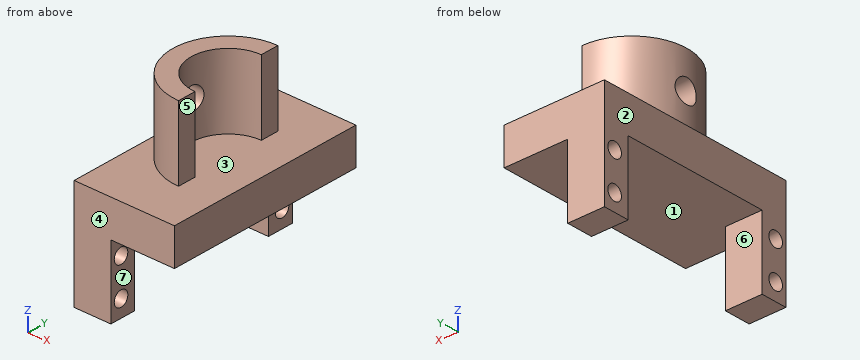
from build123d import *

# Parameters (mm, degrees)
BOSS_EXTRUDE1_DEPTH = 19.812
SKETCH2_R           = 3.175
CUT_EXTRUDE2_DEPTH  = 29.880704735
SKETCH3_W           = 34.1757
SKETCH3_H           = 54.2544
BOSS_EXTRUDE2_DEPTH = 9.906
SKETCH4_W           = 9.906
SKETCH4_H           = 7.112
BOSS_EXTRUDE3_DEPTH = 19.4691
SKETCH5_R           = 2.032
CUT_EXTRUDE3_DEPTH  = 53.599999528
SKETCH6_W           = 7.112
SKETCH6_H           = 54.2544
CUT_EXTRUDE4_DEPTH  = 44.715433515


with BuildPart() as part:
    # Sketch1 → Boss-Extrude1 (new body)
    with BuildSketch(Plane.XY):
        with BuildLine():
            Line((0, 14.859), (0, 9.906))
            ThreePointArc((0, 9.906), (-9.906, 0), (0, -9.906))
            Line((0, -9.906), (0, -14.859))
            ThreePointArc((0, -14.859), (-14.859, 0), (0, 14.859))
        make_face()
    extrude(amount=BOSS_EXTRUDE1_DEPTH)

    # Sketch2 → Cut-Extrude2 (cut, through all)
    with BuildSketch(Plane(origin=(0, 0, 0), x_dir=(0, 0, -1), z_dir=(1, 0, 0))):
        with Locations(Location((-9.906, 0, 0), (0, 0, 90))):
            Circle(SKETCH2_R)
    extrude(amount=-CUT_EXTRUDE2_DEPTH, mode=Mode.SUBTRACT)

    # Sketch3 → Boss-Extrude2 (add)
    with BuildSketch(Plane(origin=(0, 0, 0), x_dir=(-1, 0, 0), z_dir=(0, 0, -1))):
        Rectangle(SKETCH3_W, SKETCH3_H)
    extrude(amount=BOSS_EXTRUDE2_DEPTH)

    # Sketch4 → Boss-Extrude3 (add)
    with BuildSketch(Plane(origin=(0, 0, -9.906), x_dir=(-1, 0, 0), z_dir=(0, 0, -1))):
        with Locations((12.13485, -23.5712)):
            Rectangle(SKETCH4_W, SKETCH4_H)
        with Locations((12.13485, 23.5712)):
            Rectangle(SKETCH4_W, SKETCH4_H)
    extrude(amount=BOSS_EXTRUDE3_DEPTH)

    # Sketch5 → Cut-Extrude3 (cut, through all)
    with BuildSketch(Plane.ZY.offset(17.08785)):
        with Locations((-24.8031, 24.0792)):
            Circle(SKETCH5_R)
        with Locations((-14.8971, 24.0792)):
            Circle(SKETCH5_R)
        with Locations(Location((-14.8971, -24.0792, 0), (0, 0, 270))):
            Circle(SKETCH5_R)
        with Locations(Location((-24.8031, -24.0792, 0), (0, 0, 270))):
            Circle(SKETCH5_R)
    extrude(amount=-CUT_EXTRUDE3_DEPTH, mode=Mode.SUBTRACT)

    # Sketch6 → Cut-Extrude4 (cut, through all)
    with BuildSketch(Plane(origin=(0, 0, -9.906), x_dir=(-1, 0, 0), z_dir=(0, 0, -1))):
        with Locations((-13.53185, 0)):
            Rectangle(SKETCH6_W, SKETCH6_H)
    extrude(amount=-CUT_EXTRUDE4_DEPTH, mode=Mode.SUBTRACT)


solid = part.part
Verification items for the finished model (mm, model axes). Face numbers are marked on the shaded views. A direction names the side the tool comes from. Give positions to 0.01 mm unless a question says otherwise; leave off trailing zeros. Write each loop counter-clockwise with the first axis right and the second up, starting at its lowest first coordinate (ties: lowest second). Pieces come first, ordered by that corner, then holes. Notation, with made-up numbers: (75, 70.5) - (85, 70.5) arc R31 cw to (85, 96.5) - close; hole circle Ø7 at (76.5, 24.25). An arc over 180 degrees is marked (long way). Answer as CSV lines item,"result". Start each with the question number.
1. Depth check by flat-ended pin: pin 1 (8 mm diameter, centred on x = 3, y = 12.5, fed in from -Z); pin 2 (4 mm diameter, centred on y = -13, z = 6, fed in from +X); pin 3 (2 mm diameter, centred on y = 21.5, z = 0.5, fed in from +X); pin 4 (2 mm diameter, centred on x = 3, y = -20, fed in from +Z). Enter the tip coordinate at first touch or a pass-through.
2. Draft check along Y on the marked faces 1, 2, 3 and 4. Enter one of: pulls with the +Y half, pulls with the -Y half, needs draft (parallel to the pull), parting line crosses it, or undercut.
3. Sectioned sample at D-D (z = 8). Record the boundary of the cut face in (x, y).
4. Sectioned sample at A-A (y = 0). Record the boundary of the cut face in (x, z).
5. Sectioned sample at C-C (x = -13.5). Record the boundary of the cut face in (y, z) (3 decimals), then the cut area to 3 significant figures.
6. Thickness scan on line 1 (Y direction, x = -12, z = -26.5); line 2 (Z direction, x = -15.5, y = 23); line 3 (Y direction, x = -7.5, z = -11). Record the ranges inside material, lowest first.
7. Set-up check for the marked faces 5, 6 and 7: record each of +Z, -Z, +X, -X, +Y, -Y from which the full face is reachable in a straight line by a thin tool's end or side.
8. Sectioned sample at B-B (z = -11). Record the boundary of the cut face in (x, y).
Derived:
1,pin 1,"z = -9.91"
1,pin 2,"x = 0"
1,pin 3,"x = 9.98"
1,pin 4,"z = 0"
2,face 1,"undercut"
2,face 2,"needs draft"
2,face 3,"undercut"
2,face 4,"pulls with the -Y half"
3,outline,"(-14.64, -2.54) arc R14.86 ccw to (0, -14.86) - (0, -9.91) arc R9.91 cw to (-9.58, -2.54) - close; (-14.64, 2.54) - (-9.58, 2.54) arc R9.91 cw to (0, 9.91) - (0, 14.86) arc R14.86 ccw to start"
4,outline,"(-17.09, -9.91) - (9.98, -9.91) - (9.98, 0) - (-9.91, 0) - (-9.91, 6.73) - (-14.86, 6.73) - (-14.86, 0) - (-17.09, 0) - close; (-14.86, 13.08) - (-9.91, 13.08) - (-9.91, 19.81) - (-14.86, 19.81) - close"
5,outline,"(-27.127, -29.375) - (-20.015, -29.375) - (-20.015, -9.906) - (20.015, -9.906) - (20.015, -29.375) - (27.127, -29.375) - (27.127, 0) - (6.208, 0) - (6.208, 19.812) - (-6.208, 19.812) - (-6.208, 0) - (-27.127, 0) - close; hole circle Ø4.064 at (-24.079, -24.803); hole circle Ø4.064 at (-24.079, -14.897); hole circle Ø6.35 at (0, 9.906); hole circle Ø4.064 at (24.079, -24.803); hole circle Ø4.064 at (24.079, -14.897)"
5,area,"977 mm²"
6,line 1,"-27.13 to -25.2, -22.96 to -20.02, 20.02 to 22.96, 25.2 to 27.13"
6,line 2,"-29.38 to -26.52, -23.08 to -16.62, -13.18 to 0"
6,line 3,"-27.13 to -20.02, 20.02 to 27.13"
7,face 5,"+Z, +X, +Y, -Y"
7,face 6,"-Z, +X, -X"
7,face 7,"-Z, +X, +Y, -Y"
8,outline,"(-17.09, -27.13) - (-7.18, -27.13) - (-7.18, -20.02) - (-17.09, -20.02) - close; (-17.09, 20.02) - (-7.18, 20.02) - (-7.18, 27.13) - (-17.09, 27.13) - close"
